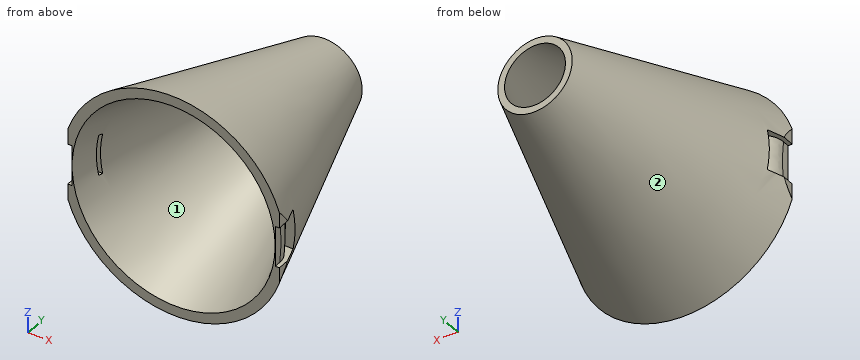
Autodesk Inventor part; units mm, degrees
ref_plane "YZ Plane" through (0, 0, 0) normal (1, 0, 0) x (0, 1, 0)
ref_plane "XZ Plane" through (0, 0, 0) normal (0, 1, 0) x (-1, 0, 0)
ref_plane "XY Plane" through (0, 0, 0) normal (0, 0, 1) x (1, 0, 0)
sketch "Sketch1" plane through (0, 0, 0) normal (0, 1, 0) x (-1, 0, 0)
  point P0 (0, 0)
sketch "Sketch2" plane through (0, 0, 0) normal (0, 1, 0) x (-1, 0, 0)
  circle A0 centre (0, 0) radius 7.5
  dimension "d0" = 15
extrude "Extrusion1" add sketch "Sketch2" along normal blind 60
sketch "Sketch3" plane through (0, 60, 0) normal (0, 1, 0) x (1, 0, 0)
  circle A0 centre (0, 0) radius 7.5
sketch "Sketch4" plane through (0, 0, 0) normal (0, -1, 0) x (1, 0, 0)
  circle A0 centre (0, 0) radius 25
  circle A1 centre (0, 0) radius 7.5
  circle A2 centre (0, 0) radius 27.5
  dimension "d3" = 50
  dimension "d4" = 55
loft "Loft1" add profiles "Sketch4" section 1 edges at (7.5, 60, 0) contours A0 | A1 | A2
sketch "Sketch5" plane through (0, 0, 0) normal (0, -1, 0) x (1, 0, 0)
  circle A0 centre (0, 0) radius 7.5
  circle A1 centre (0, 0) radius 27.5
  circle A2 centre (0, 0) radius 25
  circle A3 centre (0, 0) radius 7.5
  dimension "d9" = 50
  dimension "d10" = 15
sketch "Sketch6" plane through (0, 60, 0) normal (0, 1, 0) x (1, 0, 0)
  circle A0 centre (0, 0) radius 7.5
extrude "Extrusion2" cut sketch "Sketch6" against normal blind 5
sketch "Sketch7" plane through (0, 55, 0) normal (0, 1, 0) x (1, 0, 0)
  circle A0 centre (0, 0) radius 7.5
  line L0 (-11.197, -10.4421) -> (10.2744, -10.4421)
  line L1 (10.2744, -10.4421) -> (10.2744, 11.5325)
  line L2 (10.2744, 11.5325) -> (-11.197, 11.5325)
  line L3 (-11.197, 11.5325) -> (-11.197, -10.4421)
loft "Loft2" cut profiles "Sketch5" section 1 edges at (-7.5, 55, 0) contours A0 | A2
extrude "Extrusion3" cut sketch "Sketch7" along normal through all
sketch "Sketch8" plane through (0, 0, 0) normal (0, -1, 0) x (1, 0, 0)
  circle A0 centre (0, 0) radius 25
  circle A1 centre (0, 0) radius 27.5
  line L0 (27.5, 0) -> (27.5, -5)
  line L1 (27.0416, -5) -> (26.0416, -5)
  line L2 (26.0416, -5) -> (26.0416, 5)
  line L3 (26.0416, 5) -> (27.0416, 5)
  line L4 (27.0416, 5) -> (27.0416, -5)
  line L5 (-27.5, 0) -> (-27.5, -5)
  line L6 (-27.0416, -5) -> (-26.0416, -5)
  line L7 (-26.0416, -5) -> (-26.0416, 5)
  line L8 (-26.0416, 5) -> (-27.0416, 5)
  line L9 (-27.0416, 5) -> (-27.0416, -5)
  line L10 (26.0416, -5) -> (25.0416, -5)
  line L11 (25.0416, -5) -> (25.0416, 5)
  line L12 (25.0416, 5) -> (26.0416, 5)
  line L13 (26.0416, 5) -> (26.0416, -5)
  line L14 (-26.0416, -5) -> (-25.0416, -5)
  line L15 (-25.0416, -5) -> (-25.0416, 5)
  line L16 (-25.0416, 5) -> (-26.0416, 5)
  line L17 (-26.0416, 5) -> (-26.0416, -5)
  line L18 (-26.0416, 5) -> (-26.0416, 8.8365)
  line L19 (-26.0416, -5) -> (-26.0416, -8.8365)
  line L20 (26.0416, -5) -> (26.0416, -8.8365)
  line L21 (26.0416, 5) -> (26.0416, 8.8365)
  circle A2 centre (0, 0) radius 27.5
  dimension "d19" = 5
  dimension "d20" = 1
  dimension "d21" = 10
  dimension "d22" = 5
  dimension "d23" = 1
  dimension "d24" = 10
  dimension "d25" = 1
  dimension "d26" = 1
extrude "Extrusion4" cut sketch "Sketch8" against normal through all contours A1 L4 | L3 L21 A1 | L4 L1 L2 L3 | A1 L20 L1 | L18 L8 A1 | A1 L6 L19 | L9 A1 | L8 L7 L6 L9
sketch "Sketch9" plane through (0, 0, 0) normal (0, -1, 0) x (1, 0, 0)
  circle A0 centre (0, 0) radius 27.5
  circle A1 centre (0, 0) radius 25
  line L0 (27.5, 0) -> (27.5, -5)
  line L1 (26.0416, -8.8365) -> (26.0416, 8.8365)
  line L2 (27.0416, -5) -> (26.0416, -5)
  line L3 (26.0416, -5) -> (26.0416, 5)
  line L4 (26.0416, 5) -> (27.0416, 5)
  line L5 (27.0416, 5) -> (27.0416, -5)
  line L6 (26.0416, 5) -> (25.0416, 5)
  line L7 (25.0416, 5) -> (25.0416, -5)
  line L8 (25.0416, -5) -> (26.0416, -5)
  line L9 (26.0416, -5) -> (26.0416, 5)
  line L10 (-27.5, 0) -> (-27.5, -5)
  line L11 (-26.0416, 8.8365) -> (-26.0416, -8.8365)
  line L12 (-27.0416, -5) -> (-26.0416, -5)
  line L13 (-26.0416, -5) -> (-26.0416, 5)
  line L14 (-26.0416, 5) -> (-27.0416, 5)
  line L15 (-27.0416, 5) -> (-27.0416, -5)
  line L16 (-26.0416, -5) -> (-25.0416, -5)
  line L17 (-25.0416, -5) -> (-25.0416, 5)
  line L18 (-25.0416, 5) -> (-26.0416, 5)
  line L19 (-26.0416, 5) -> (-26.0416, -5)
  dimension "d29" = 5
  dimension "d30" = 10
  dimension "d31" = 1
  dimension "d32" = 5
  dimension "d33" = 10
  dimension "d34" = 1
extrude "Extrusion5" cut sketch "Sketch9" against normal blind 7 contours L1 L8 L7 L6 | L18 L17 L16 L11
sketch "Sketch10" plane through (25.0416, 0, 5) normal (1, 0, 0) x (0, 0, -1)
  line L0 (0, 0) -> (10, 0)
  line L1 (10, 0) -> (10, 7)
  line L2 (10, 7) -> (0, 7)
  line L3 (0, 7) -> (0, 0)
  line L4 (10, 7) -> (0, 7)
  line L5 (0, 7) -> (0, 6)
  line L6 (0, 6) -> (10, 6)
  line L7 (10, 6) -> (10, 7)
  point P0 (5, 0)
  dimension "d37" = 10
  dimension "d38" = 7
  dimension "d39" = 1
extrude "Extrusion6" cut sketch "Sketch10" against normal through all contours L3 L2 L1 L6
fillet "Fillet1" radius 5 1 edges at (25.0416, 6, 0)
fillet "Fillet2" radius 5 1 edges at (-25.0416, 6, 0)
properties part number "cone_p2_testpart1"
Check sheet for the modelled part. Datum: model origin and axes. Units: mm. Face numbers are marked on the shaded views. Round coordinates to 2 decimals unless told otherwise and drop trailing zeros. Loops run counter-clockwise (first coordinate to the right, second up) from the corner with the lowest first, then second, coordinate; pieces in that order, holes last. Notation, with made-up numbers: (16.25, -18) - (40.25, -18) arc R24 cw to (40.25, 18) - close; hole circle Ø10 at (31.25, 73). An arc over 180 degrees is marked (long way). Write item = value, one per line. Start each with the question number.
Q1. Release check for a two-part mould opening along X. For the marked faces 1 and 2 record: pulls with the +X half, pulls with the -X half, needs draft (parallel to the pull), parting line crosses it, or undercut.
Q2. Section check B-B (z = 0). Count the separate pieces of the cut face and the enclosed holes in it, plus the area to 3 significant figures.
Q3. Section check D-D (y = 12.5). Record the boundary of the cut face in (x, z).
Q4. Depth check by flat-ended pin: P1, Ø1, axis at y = 1, z = 2, coming from the +X side; P2, Ø3, axis at x = -23.5, y = 3, coming from the +Z side; P3, Ø4, axis at y = 19.5, z = 19, coming from the +X side. Enter the tip coordinate at first touch or a pass-through.
Q5. Thickness scan on L1, parallel to X at y = 20, z = -16; L2, parallel to X at y = 13.5, z = 0.5; L3, parallel to Z at x = -4, y = 39. Record the ranges inside material, lowest first.
Q6. Section check C-C (y = 25). Record the boundary of the cut face in (x, z), plus the area to 3 significant figures.
Q7. Section check A-A (x = 0). Record the boundary of the cut face in (y, z), plus the area to 3 significant figures.
Derived:
q1.face_1 = undercut
q1.face_2 = parting line crosses it
q2.separate_pieces = 4
q2.enclosed_holes = 0
q2.area = 202 mm^2
q3.outline = circle Ø46.67 at (0, 0); hole circle Ø42.05 at (0, 0)
q4.P1 = 25.04
q4.P2 = 14.95
q4.P3 = 12.55
q5.L1 = -13.34 to -9.56, 9.56 to 13.34
q5.L2 = -22.99 to -20.7, 20.7 to 22.99
q5.L3 = -13.94 to -11.94, 11.94 to 13.94
q6.outline = circle Ø38.33 at (0, 0); hole circle Ø34.09 at (0, 0)
q6.area = 241 mm^2
q7.outline = (0, -27.5) - (55, -9.17) - (55, -7.5) - (0, -25) - close; (0, 25) - (55, 7.5) - (55, 9.17) - (0, 27.5) - close
q7.area = 229 mm^2
